Work out the finished part from the listing and answer in its coordinate system (mm). Face numbers are marked on the shaded views. A direction names the side the tool comes from. Coordinates: 2 decimals unless noted, no trailing zeros. Order: outer loops, then holes, each group sorted by start corner. A loop starts at its lowest first (then second) coordinate and runs counter-clockwise, first axis right, second up. Notation, with made-up numbers: M 61,-6 L 85,-6 A10 ccw 85,11 Z; hole C 75.25,88 d10. An arc over 180 degrees is marked long. Answer in a Markdown table with one row per item. Add a question column.
Item 1: The part is cut by section C-C (y = 8.25). Write down the section's boundary in (x, z) (3 decimals).
Item 2: Which of the six approach directions +Z, -Z, +X, -X, +Y, -Y give full straight-line access (tool end or side, diameter ignored) to the marked faces 5, 6, 7 and 8?
Item 3: The part is cut by section B-B (x = 18.5). Write down the section's boundary in (y, z), then the cut area to 3 significant figures.
Item 4: The mould has two halves that part along X. Classify the marked faces 1, 2, 3 and 4: released by +X, released by -X, zero draft, split by the parting line, or undercut.
Item 5: Consider line 1 (Z direction, x = 18.5, y = 3.5); line 2 (X direction, y = 6.75, z = -11.5); line 3 (X direction, y = 5, z = -11.5). Determine where each line is inside the solid, lowest interval first. Write a range as from..to.
Item 6: The part is cut by section A-A (x = 9). Write down the section's boundary in (y, z), then the cut area to 3 significant figures.
Item 7: The part is cut by section D-D (z = -11.5). Write down the section's boundary in (x, y).
Item 8: Flat-ended cylindrical pins translate along their axes: pin 1 Ø5 at (y, z) = (6, 1.5) entering from +X; pin 2 Ø8 at (y, z) = (16.5, -3) entering from +X; pin 3 Ø5 at (y, z) = (2.5, 0.5) entering from +X. Find the tip coordinate at first contact, or state that the pin passes through.
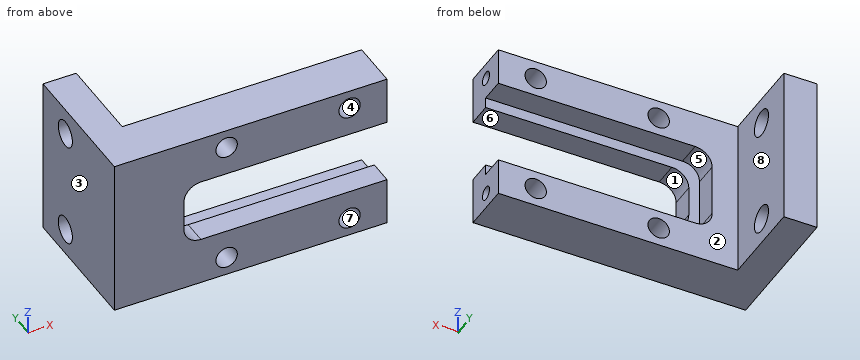
from build123d import *

# Parameters (mm, degrees)
SKETCH1_W                    = 51
SKETCH1_H                    = 30
BOSS_EXTRUDE1_DEPTH          = 9
SKETCH2_W                    = 6.21
SKETCH2_H                    = 30
BOSS_EXTRUDE2_DEPTH          = 16.38
SKETCH3_W                    = 40
SKETCH3_H                    = 16
CUT_EXTRUDE1_DEPTH           = 4.5
FILLET1_R                    = 3.175
CUT_EXTRUDE2_DEPTH           = 37.210832633
F_5_0_5_DIAMETER_HOLE1_D     = 5
F_5_0_5_DIAMETER_HOLE1_DEPTH = 10
F_5_0_5_DIAMETER_HOLE1_TIP   = 1.502151548
F_4_0_4_DIAMETER_HOLE1_D     = 4
F_4_0_4_DIAMETER_HOLE1_DEPTH = 10
F_4_0_4_DIAMETER_HOLE1_TIP   = 1.201721238
M3X0_5_TAPPED_HOLE1_D        = 2.5
M3X0_5_TAPPED_HOLE1_DEPTH    = 7
M3X0_5_TAPPED_HOLE1_TIP      = 0.751075774


with BuildPart() as part:
    # Sketch1 → Boss-Extrude1 (new body)
    with BuildSketch(Plane(origin=(0, 0, 0), x_dir=(1, 0, 0), z_dir=(0, 1, 0))):
        Rectangle(SKETCH1_W, SKETCH1_H)
    extrude(amount=BOSS_EXTRUDE1_DEPTH)

    # Sketch2 → Boss-Extrude2 (add)
    with BuildSketch(Plane(origin=(0, 9, 0), x_dir=(1, 0, 0), z_dir=(0, 1, 0))):
        with Locations((-22.395, 0)):
            Rectangle(SKETCH2_W, SKETCH2_H)
    extrude(amount=BOSS_EXTRUDE2_DEPTH)

    # Sketch3 → Cut-Extrude1 (cut)
    with BuildSketch(Plane(origin=(0, 9, 0), x_dir=(1, 0, 0), z_dir=(0, 1, 0))):
        with Locations((5.5, 0)):
            Rectangle(SKETCH3_W, SKETCH3_H)
    extrude(amount=-CUT_EXTRUDE1_DEPTH, mode=Mode.SUBTRACT)

    # Fillet1
    fillet1_edges = [part.edges().sort_by_distance(p)[0] for p in [
        (-14.5, 6.75, 8),
        (-14.5, 6.75, -8),
    ]]
    fillet(fillet1_edges, radius=FILLET1_R)

    # Sketch5 → Cut-Extrude2 (cut, through all)
    with BuildSketch(Plane(origin=(0, 4.5, 0), x_dir=(1, 0, 0), z_dir=(0, 1, 0))):
        with BuildLine():
            Line((25.5, -6), (-9.325, -6))
            ThreePointArc((-9.325, -6), (-11.57006403, -5.07006403), (-12.5, -2.825))
            Line((-12.5, -2.825), (-12.5, 2.825))
            ThreePointArc((-12.5, 2.825), (-11.57006403, 5.07006403), (-9.325, 6))
            Line((-9.325, 6), (25.5, 6))
            Line((25.5, 6), (25.5, -6))
        make_face()
    extrude(amount=-CUT_EXTRUDE2_DEPTH, mode=Mode.SUBTRACT)

    # Ø5.0 (5) Diameter Hole1
    with Locations(Plane(origin=(-19.29, 0, 0), x_dir=(0, 0, -1), z_dir=(1, 0, 0))):
        with Locations((-10, 17.432129573), (10, 17.432129573)):
            Hole(F_5_0_5_DIAMETER_HOLE1_D / 2, depth=F_5_0_5_DIAMETER_HOLE1_DEPTH)
            with Locations((0, 0, -(F_5_0_5_DIAMETER_HOLE1_DEPTH + F_5_0_5_DIAMETER_HOLE1_TIP / 2))):  # 118° drill point
                Cone(0, F_5_0_5_DIAMETER_HOLE1_D / 2, F_5_0_5_DIAMETER_HOLE1_TIP, mode=Mode.SUBTRACT)

    # Ø4.0 (4) Diameter Hole1
    with Locations(Plane(origin=(0, 9, 0), x_dir=(1, 0, 0), z_dir=(0, 1, 0))):
        with Locations((73.579545509, -261.26638596), (-4.5, -11.5), (18.5, -11.5), (18.5, 11.5), (-4.5, 11.5)):
            Hole(F_4_0_4_DIAMETER_HOLE1_D / 2, depth=F_4_0_4_DIAMETER_HOLE1_DEPTH)
            with Locations((0, 0, -(F_4_0_4_DIAMETER_HOLE1_DEPTH + F_4_0_4_DIAMETER_HOLE1_TIP / 2))):  # 118° drill point
                Cone(0, F_4_0_4_DIAMETER_HOLE1_D / 2, F_4_0_4_DIAMETER_HOLE1_TIP, mode=Mode.SUBTRACT)

    # M3x0.5 Tapped Hole1
    with Locations(Plane(origin=(25.5, 0, 0), x_dir=(0, 0, -1), z_dir=(1, 0, 0))):
        with Locations((-12, 4.623330266), (12, 4.623330266)):
            Hole(M3X0_5_TAPPED_HOLE1_D / 2, depth=M3X0_5_TAPPED_HOLE1_DEPTH)
            with Locations((0, 0, -(M3X0_5_TAPPED_HOLE1_DEPTH + M3X0_5_TAPPED_HOLE1_TIP / 2))):  # 118° drill point
                Cone(0, M3X0_5_TAPPED_HOLE1_D / 2, M3X0_5_TAPPED_HOLE1_TIP, mode=Mode.SUBTRACT)


solid = part.part
Reply:
| question | item | result |
|---|---|---|
| 1 | outline | M -25.5,-15 L 25.5,-15 L 25.5,-8 L -11.325,-8 A3.175 cw -14.5,-4.825 L -14.5,4.825 A3.175 cw -11.325,8 L 25.5,8 L 25.5,15 L -25.5,15 Z; hole C -4.5,-11.5 d4; hole C -4.5,11.5 d4; hole C 18.5,-11.5 d4; hole C 18.5,11.5 d4 |
| 2 | face 5 | +X, +Y |
| 2 | face 6 | +X, +Y, -Y |
| 2 | face 7 | +Y, -Y |
| 2 | face 8 | +Z, -Z, +X, +Y |
| 3 | outline | M 0,-15 L 9,-15 L 9,-13.5 L 0,-13.5 Z; M 0,-9.5 L 9,-9.5 L 9,-8 L 4.5,-8 L 4.5,-6 L 0,-6 Z; M 0,6 L 4.5,6 L 4.5,8 L 9,8 L 9,9.5 L 0,9.5 Z; M 0,13.5 L 9,13.5 L 9,15 L 0,15 Z |
| 3 | area | 72.0 mm2 |
| 4 | face 1 | released by +X |
| 4 | face 2 | zero draft |
| 4 | face 3 | released by -X |
| 4 | face 4 | undercut |
| 5 | line 1 | z = -15..-13.5, -9.5..-6, 6..9.5, 13.5..15 |
| 5 | line 2 | x = -25.5..-6.5, -2.5..16.5, 20.5..25.5 |
| 5 | line 3 | x = -25.5..-6.5, -2.5..16.5 |
| 6 | outline | M 0,-15 L 9,-15 L 9,-8 L 4.5,-8 L 4.5,-6 L 0,-6 Z; M 0,6 L 4.5,6 L 4.5,8 L 9,8 L 9,15 L 0,15 Z |
| 6 | area | 144 mm2 |
| 7 | outline | M -25.5,0 L -6.5,0 L -6.5,9 L -19.29,9 L -19.29,15.43 L -25.5,15.43 Z; M -25.5,19.43 L -19.29,19.43 L -19.29,25.38 L -25.5,25.38 Z; M -2.5,0 L 16.5,0 L 16.5,9 L -2.5,9 Z; M 20.5,0 L 25.5,0 L 25.5,3.48 L 20.5,3.48 Z; M 20.5,5.77 L 25.5,5.77 L 25.5,9 L 20.5,9 Z |
| 8 | pin 1 | stops at x = -12.43 |
| 8 | pin 2 | stops at x = -19.29 |
| 8 | pin 3 | stops at x = -12.5 |
